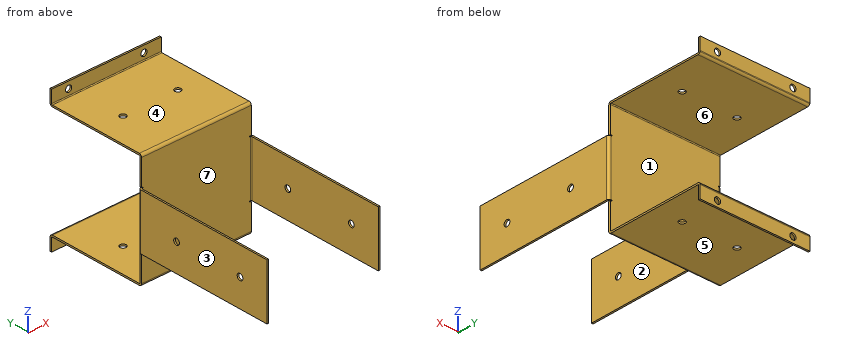
```python
from build123d import *

# Parameters (mm, degrees)
BASE_FLANGE1_DEPTH              = 50.8
EDGE_FLANGE1_STRIP_W            = 7.59968
EDGE_FLANGE1_STRIP_H            = 1.51892
EDGE_FLANGE1_STRIP_CUT_DEPTH    = 50.8
EDGE_FLANGE1_RELIEF_W           = 8.35914
EDGE_FLANGE1_RELIEF_H           = 0.75946
EDGE_FLANGE1_RELIEF_CUT_DEPTH   = 1.51892
EDGE_FLANGE1_STRIP_2_W          = 7.59968
EDGE_FLANGE1_STRIP_2_H          = 1.51892
EDGE_FLANGE1_STRIP_CUT_2_DEPTH  = 50.8
EDGE_FLANGE1_RELIEF_2_W         = 8.35914
EDGE_FLANGE1_RELIEF_2_H         = 0.75946
EDGE_FLANGE1_RELIEF_CUT_2_DEPTH = 1.51892
EDGE_FLANGE1_DEPTH              = 50.8
EDGE_FLANGE1_BEND_DEPTH         = 50.8
SKETCHED_START                  = -50.8
SKETCHED_BEND1_DEPTH            = 101.6
SKETCHED_BEND1_2_DEPTH          = 101.6
SKETCHED_BEND2_DEPTH            = 101.6
SKETCHED_BEND2_2_DEPTH          = 101.6
SKETCH15_R                      = 2.8575
CUT_EXTRUDE1_DEPTH              = 178.869439856
SKETCH17_R                      = 2.8575
CUT_EXTRUDE2_DEPTH              = 2.54
SKETCH18_R                      = 2.8575
CUT_EXTRUDE3_DEPTH              = 182.441822775


# Read off the part's stored shape, not the designer's step: Sketched Bend1, Sketched Bend2
# Sheet-metal steps are written as plain solids
with BuildPart() as part:
    # Sketch2 → Base-Flange1 (new, symmetric)
    with BuildSketch(Plane(origin=(0, 0, 0), x_dir=(0, 0, -1), z_dir=(1, 0, 0))):
        with BuildLine():
            Line((-50.8, 101.6), (-50.8, 0.762))
            ThreePointArc((-50.8, 0.762), (-50.576815367, 0.223184633), (-50.038, 0))
            Line((-50.038, 0), (50.038, 0))
            ThreePointArc((50.038, 0), (50.576815367, 0.223184633), (50.8, 0.762))
            Line((50.8, 0.762), (50.8, 101.6))
            Line((50.8, 101.6), (52.31892, 101.6))
            Line((52.31892, 101.6), (52.31892, 0.762))
            ThreePointArc((52.31892, 0.762), (51.650853999, -0.850853999), (50.038, -1.51892))
            Line((50.038, -1.51892), (-50.038, -1.51892))
            ThreePointArc((-50.038, -1.51892), (-51.650853999, -0.850853999), (-52.31892, 0.762))
            Line((-52.31892, 0.762), (-52.31892, 101.6))
            Line((-52.31892, 101.6), (-50.8, 101.6))
        make_face()
    extrude(amount=BASE_FLANGE1_DEPTH, both=True)

    # Edge-Flange1 strip (across the edge) → Edge-Flange1 strip cut (cut)
    with BuildSketch(Plane(origin=(50.8, -1.51892, -25.4), x_dir=(-1, 0, 0), z_dir=(0, 0, 1))):
        with Locations((-3.03784, -0.75946)):
            Rectangle(EDGE_FLANGE1_STRIP_W, EDGE_FLANGE1_STRIP_H)
    extrude(amount=EDGE_FLANGE1_STRIP_CUT_DEPTH, mode=Mode.SUBTRACT)

    # Edge-Flange1 relief (on the sheet) → Edge-Flange1 relief cut (cut)
    with BuildSketch(Plane(origin=(50.038, -1.51892, -25.4), x_dir=(-1, 0, 0), z_dir=(0, -1, 0))):
        with Locations((-3.42011, 0.37973)):
            Rectangle(EDGE_FLANGE1_RELIEF_W, EDGE_FLANGE1_RELIEF_H)
        with Locations((-3.42011, -51.17973)):
            Rectangle(EDGE_FLANGE1_RELIEF_W, EDGE_FLANGE1_RELIEF_H)
    extrude(amount=-EDGE_FLANGE1_RELIEF_CUT_DEPTH, mode=Mode.SUBTRACT)

    # Edge-Flange1 strip 2 (across the edge) → Edge-Flange1 strip cut 2 (cut)
    with BuildSketch(Plane(origin=(-50.8, -1.51892, 25.4), x_dir=(1, 0, 0), z_dir=(0, 0, -1))):
        with Locations((-3.03784, -0.75946)):
            Rectangle(EDGE_FLANGE1_STRIP_2_W, EDGE_FLANGE1_STRIP_2_H)
    extrude(amount=EDGE_FLANGE1_STRIP_CUT_2_DEPTH, mode=Mode.SUBTRACT)

    # Edge-Flange1 relief 2 (on the sheet) → Edge-Flange1 relief cut 2 (cut)
    with BuildSketch(Plane(origin=(-50.038, -1.51892, 25.4), x_dir=(1, 0, 0), z_dir=(0, -1, 0))):
        with Locations((-3.42011, 0.37973)):
            Rectangle(EDGE_FLANGE1_RELIEF_2_W, EDGE_FLANGE1_RELIEF_2_H)
        with Locations((-3.42011, -51.17973)):
            Rectangle(EDGE_FLANGE1_RELIEF_2_W, EDGE_FLANGE1_RELIEF_2_H)
    extrude(amount=-EDGE_FLANGE1_RELIEF_CUT_2_DEPTH, mode=Mode.SUBTRACT)

    # Edge-Flange1 section (across the edge) → Edge-Flange1 (add)
    with BuildSketch(Plane(origin=(50.8, -1.51892, -25.4), x_dir=(-1, 0, 0), z_dir=(0, 0, 1))):
        with BuildLine():
            Line((-1.51892, 0.762), (-1.51892, 127))
            Line((-1.51892, 127), (0, 127))
            Line((0, 127), (0, 0.762))
            ThreePointArc((0, 0.762), (0.223184633, 0.223184633), (0.762, 0))
            Line((0.762, 0), (0.762, -1.51892))
            ThreePointArc((0.762, -1.51892), (-0.850853999, -0.850853999), (-1.51892, 0.762))
        make_face()
    extrude(amount=EDGE_FLANGE1_DEPTH)

    # Edge-Flange1 section 2 (across the edge) → Edge-Flange1 bend (add)
    with BuildSketch(Plane(origin=(-50.8, -1.51892, 25.4), x_dir=(1, 0, 0), z_dir=(0, 0, -1))):
        with BuildLine():
            Line((-1.51892, 0.762), (-1.51892, 127))
            Line((-1.51892, 127), (0, 127))
            Line((0, 127), (0, 0.762))
            ThreePointArc((0, 0.762), (0.223184633, 0.223184633), (0.762, 0))
            Line((0.762, 0), (0.762, -1.51892))
            ThreePointArc((0.762, -1.51892), (-0.850853999, -0.850853999), (-1.51892, 0.762))
        make_face()
    extrude(amount=EDGE_FLANGE1_BEND_DEPTH)

    # Sketched Bend1 outline → Sketched Bend1 (cut)
    with BuildSketch(Plane.YZ.offset(SKETCHED_START)):
        with BuildLine():
            ThreePointArc((89.854920675, 52.31892), (89.021204447, 51.218038215), (87.70504811, 50.8))
            Line((87.70504811, 50.8), (101.6, 50.8))
            Line((101.6, 50.8), (101.6, 52.31892))
            Line((101.6, 52.31892), (89.854920675, 52.31892))
        make_face()
    extrude(amount=SKETCHED_BEND1_DEPTH, mode=Mode.SUBTRACT)

    # Sketched Bend1 2 outline → Sketched Bend1 2 (add)
    with BuildSketch(Plane.YZ.offset(SKETCHED_START)):
        with BuildLine():
            Line((87.70504811, 52.31892), (89.854920675, 52.31892))
            ThreePointArc((89.854920675, 52.31892), (89.952967523, 52.694326729), (89.98596811, 53.08092))
            Line((89.98596811, 53.08092), (89.98596811, 64.58596811))
            Line((89.98596811, 64.58596811), (88.46704811, 64.58596811))
            Line((88.46704811, 64.58596811), (88.46704811, 53.08092))
            ThreePointArc((88.46704811, 53.08092), (88.243863477, 52.542104633), (87.70504811, 52.31892))
        make_face()
    extrude(amount=SKETCHED_BEND1_2_DEPTH)

    # Sketched Bend2 outline → Sketched Bend2 (cut)
    with BuildSketch(Plane.YZ.offset(SKETCHED_START)):
        with BuildLine():
            ThreePointArc((87.70504811, -50.8), (89.021204447, -51.218038215), (89.854920675, -52.31892))
            Line((89.854920675, -52.31892), (101.6, -52.31892))
            Line((101.6, -52.31892), (101.6, -50.8))
            Line((101.6, -50.8), (87.70504811, -50.8))
        make_face()
    extrude(amount=SKETCHED_BEND2_DEPTH, mode=Mode.SUBTRACT)

    # Sketched Bend2 2 outline → Sketched Bend2 2 (add)
    with BuildSketch(Plane.YZ.offset(SKETCHED_START)):
        with BuildLine():
            Line((88.46704811, -64.58596811), (89.98596811, -64.58596811))
            Line((89.98596811, -64.58596811), (89.98596811, -53.08092))
            ThreePointArc((89.98596811, -53.08092), (89.952967523, -52.694326729), (89.854920675, -52.31892))
            Line((89.854920675, -52.31892), (87.70504811, -52.31892))
            ThreePointArc((87.70504811, -52.31892), (88.243863477, -52.542104633), (88.46704811, -53.08092))
            Line((88.46704811, -53.08092), (88.46704811, -64.58596811))
        make_face()
    extrude(amount=SKETCHED_BEND2_2_DEPTH)

    # Sketch15 → Cut-Extrude1 (cut, through all)
    with BuildSketch(Plane(origin=(52.31892, 0, 0), x_dir=(0, 0, -1), z_dir=(1, 0, 0))):
        with Locations(Location((0, -38.1, 0), (0, 0, 90))):
            Circle(SKETCH15_R)
        with Locations(Location((0, -101.6, 0), (0, 0, 90))):
            Circle(SKETCH15_R)
    extrude(amount=-CUT_EXTRUDE1_DEPTH, mode=Mode.SUBTRACT)

    # Sketch17 → Cut-Extrude2 (cut)
    with BuildSketch(Plane(origin=(0, 89.98596811, 0), x_dir=(1, 0, 0), z_dir=(0, 1, 0))):
        with Locations(Location((-35.052, 59.305404319, 0), (0, 0, 270))):
            Circle(SKETCH17_R)
        with Locations(Location((34.798, 59.305404319, 0), (0, 0, 270))):
            Circle(SKETCH17_R)
        with Locations(Location((-35.052, -58.440894052, 0), (0, 0, 270))):
            Circle(SKETCH17_R)
        with Locations(Location((34.798, -58.440894052, 0), (0, 0, 270))):
            Circle(SKETCH17_R)
    extrude(amount=-CUT_EXTRUDE2_DEPTH, mode=Mode.SUBTRACT)

    # Sketch18 → Cut-Extrude3 (cut, through all)
    with BuildSketch(Plane.XY.offset(52.31892)):
        with Locations((-25.4, 44.45)):
            Circle(SKETCH18_R)
        with Locations((25.4, 44.45)):
            Circle(SKETCH18_R)
    extrude(amount=-CUT_EXTRUDE3_DEPTH, mode=Mode.SUBTRACT)


solid = part.part
```
Input: part model. Units: mm. Frame: model coordinates. Face numbers are marked on the shaded views. A direction names the side the tool comes from. Coordinates: 2 decimals unless noted, no trailing zeros. Loops run counter-clockwise (first coordinate to the right, second up) from the corner with the lowest first, then second, coordinate; pieces in that order, holes last. Notation, with made-up numbers: (45, 73) - (53, 73) arc R16 cw to (53, 82) - close; hole circle Ø4 at (43.5, -30.75). An arc over 180 degrees is marked (long way). Answer in a Markdown table with one row per item.
(1) Pin query (flat end, axial travel): P1, Ø12.5, axis at x = 1.5, z = -57.5, coming from the -Y side; P2, Ø5, axis at x = 1, z = 45.5, coming from the +Y side; P3, Ø2.5, axis at x = 51.5, y = -60, coming from the -Z side. Return the tip coordinate at first contact, or that it passes through.
Model answer:
| item | result |
|---|---|
| P1 | stops at y = -1.17 |
| P2 | stops at y = 0 |
| P3 | stops at z = -25.4 |
(2) Cut plane D-D on y = 8. Output: boundary loops of the cut face in (x, z), plus the area to 3 significant figures.
Model answer:
| item | result |
|---|---|
| outline | (-50.8, -52.32) - (50.8, -52.32) - (50.8, -50.8) - (-50.8, -50.8) - close; (-50.8, 50.8) - (50.8, 50.8) - (50.8, 52.32) - (-50.8, 52.32) - close |
| area | 309 mm² |
(3) Material intervals for L1, parallel to Z at x = -20.5, y = 13; L2, parallel to Y at x = -4, z = -40.5, sorted ascending. Write a range as from..to.
Model answer:
| item | result |
|---|---|
| L1 | z = -52.32..-50.8, 50.8..52.32 |
| L2 | y = -1.52..0 |
(4) Set-up query: the marked faces 1, 2, 3 and 4. Return all of +Z, -Z, +X, -X, +Y, -Y with unobstructed straight access to the full face (end or side cutting, diameter ignored); none if empty.
Model answer:
| item | result |
|---|---|
| face 1 | +X, -X, +Y |
| face 2 | +Z, -Z, -Y |
| face 3 | +Z, -Z, -X, +Y, -Y |
| face 4 | +Z, +X, -X, -Y |
(5) Cut plane A-A on z = 0. Output: boundary loops of the cut face in (x, y).
Model answer:
| item | result |
|---|---|
| outline | (-52.32, -128.52) - (-50.8, -128.52) - (-50.8, -104.46) - (-52.32, -104.46) - close; (-52.32, -98.74) - (-50.8, -98.74) - (-50.8, -40.96) - (-52.32, -40.96) - close; (-52.32, -35.24) - (-50.8, -35.24) - (-50.8, -2.28) arc R0.76 cw to (-50.04, -1.52) - (50.04, -1.52) arc R0.76 cw to (50.8, -2.28) - (50.8, -35.24) - (52.32, -35.24) - (52.32, -2.28) arc R2.28 ccw to (50.04, 0) - (-50.04, 0) arc R2.28 ccw to (-52.32, -2.28) - close; (50.8, -128.52) - (52.32, -128.52) - (52.32, -104.46) - (50.8, -104.46) - close; (50.8, -98.74) - (52.32, -98.74) - (52.32, -40.96) - (50.8, -40.96) - close |
(6) Cut plane C-C on x = -25.4. Output: boundary loops of the cut face in (y, z).
Model answer:
| item | result |
|---|---|
| outline | (-1.52, -50.04) arc R2.28 ccw to (0.76, -52.32) - (41.59, -52.32) - (41.59, -50.8) - (0.76, -50.8) arc R0.76 cw to (0, -50.04) - (0, 50.04) arc R0.76 cw to (0.76, 50.8) - (41.59, 50.8) - (41.59, 52.32) - (0.76, 52.32) arc R2.28 ccw to (-1.52, 50.04) - close; (47.31, -52.32) - (87.71, -52.32) arc R0.76 cw to (88.47, -53.08) - (88.47, -64.59) - (89.99, -64.59) - (89.99, -53.08) arc R2.28 ccw to (87.71, -50.8) - (47.31, -50.8) - close; (47.31, 50.8) - (87.71, 50.8) arc R2.28 ccw to (89.99, 53.08) - (89.99, 64.59) - (88.47, 64.59) - (88.47, 53.08) arc R0.76 cw to (87.71, 52.32) - (47.31, 52.32) - close |
(7) Cut plane B-B on y = 44.45. Output: boundary loops of the cut face in (x, z), plus the area to 3 significant figures.
Model answer:
| item | result |
|---|---|
| outline | (-50.8, -52.32) - (-28.26, -52.32) - (-28.26, -50.8) - (-50.8, -50.8) - close; (-50.8, 50.8) - (-28.26, 50.8) - (-28.26, 52.32) - (-50.8, 52.32) - close; (-22.54, -52.32) - (22.54, -52.32) - (22.54, -50.8) - (-22.54, -50.8) - close; (-22.54, 50.8) - (22.54, 50.8) - (22.54, 52.32) - (-22.54, 52.32) - close; (28.26, -52.32) - (50.8, -52.32) - (50.8, -50.8) - (28.26, -50.8) - close; (28.26, 50.8) - (50.8, 50.8) - (50.8, 52.32) - (28.26, 52.32) - close |
| area | 274 mm² |
(8) Mould query, pull axis Z, two halves, no side actions, for the marked faces 5, 6 and 7. Classes: pulls with the +Z half, pulls with the -Z half, needs draft (parallel to the pull), parting line crosses it, or undercut.
Model answer:
| item | result |
|---|---|
| face 5 | pulls with the -Z half |
| face 6 | undercut |
| face 7 | needs draft |
